Input: part model. Units: mm. Frame: model coordinates. Coordinates: 2 decimals unless noted, no trailing zeros. Loops run counter-clockwise (first coordinate to the right, second up) from the corner with the lowest first, then second, coordinate; pieces in that order, holes last. Notation, with made-up numbers: (66.5, 50.5) - (75.5, 50.5) arc R13 ccw to (75.5, 61.5) - close; hole circle Ø6 at (21.25, 4.25). An arc over 180 degrees is marked (long way). Write item = value, one per line. Start each with the question number.
from build123d import *

# Parameters (mm, degrees)
SKETCH1_R           = 3.5
BOSS_EXTRUDE1_DEPTH = 6
CHAMFER1_SIZE       = 3


with BuildPart() as part:
    # Sketch1 → Boss-Extrude1 (new body)
    with BuildSketch(Plane(origin=(0, 0, 0), x_dir=(1, 0, 0), z_dir=(0, 1, 0))):
        Polygon((144, 19.194168848), (0, 19.194168848), (0, 0), (38, 0), (108, 0), (144, 0), align=None)
        with Locations(Location((108, 9.194168848, 0), (0, 0, 270))):
            Circle(SKETCH1_R, mode=Mode.SUBTRACT)
        with Locations(Location((38, 10, 0), (0, 0, 270))):
            Circle(SKETCH1_R, mode=Mode.SUBTRACT)
    extrude(amount=BOSS_EXTRUDE1_DEPTH)

    # Chamfer1
    chamfer1_edges = [part.edges().sort_by_distance(p)[0] for p in [
        (38, 0, -13.5),
        (108, 0, -12.694168848),
    ]]
    chamfer(chamfer1_edges, length=CHAMFER1_SIZE)


solid = part.part
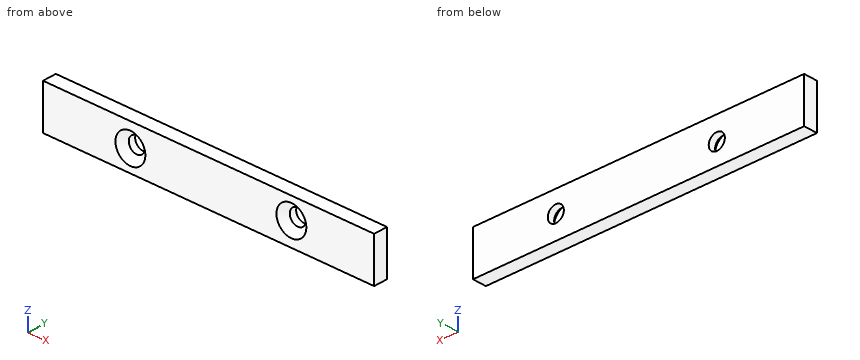
Item 1: Cut plane A-A on x = 108. Return loops of the section in (y, z).
Item 2: Cut plane C-C on z = -10. State how many separate pieces and enclosed holes the cut face has, plus the area to 3 significant figures.
Item 3: Ray query, line 1 (X direction, y = 0.7, z = -10.75); line 2 (X direction, y = 3.4, z = -7.5); line 3 (X direction, y = 4.1, z = -13). Return the intervals inside material, ascending.
Item 4: Pin query (flat end, axial travel): pin 1 (11 mm diameter, centred on x = 108, z = -9.19, fed in from -Y); pin 2 (1 mm diameter, centred on x = 95, y = 2, fed in from +Z); pin 3 (9 mm diameter, centred on x = 38, z = -10, fed in from -Y). Return the tip coordinate at first contact, or that it passes through.
Item 5: Cut plane B-B on y = 4.25. Return loops of the section in (x, z), plus the area to 3 significant figures.
Recorded:
q1.outline = (0, -19.19) - (6, -19.19) - (6, -12.69) - (3, -12.69) - (0, -15.69) - close; (0, -2.69) - (3, -5.69) - (6, -5.69) - (6, 0) - (0, 0) - close
q2.separate_pieces = 3
q2.enclosed_holes = 0
q2.area = 763 mm²
q3.line_1 = 0 to 32.25, 43.75 to 102.41, 113.59 to 144
q3.line_2 = 0 to 35.55, 40.45 to 104.94, 111.06 to 144
q3.line_3 = 0 to 36.2, 39.8 to 144
q4.pin_1 = 1
q4.pin_2 = 0
q4.pin_3 = 2
q5.outline = (0, -19.19) - (144, -19.19) - (144, 0) - (0, 0) - close; hole circle Ø7 at (38, -10); hole circle Ø7 at (108, -9.19)
q5.area = 2,690 mm²
